```python
from build123d import *

# Parameters (mm, degrees)
SKETCH2_R           = 60
BOSS_EXTRUDE2_DEPTH = 5


with BuildPart() as part:
    # Sketch2 → Boss-Extrude2 (new body)
    with BuildSketch(Plane(origin=(0, 0, 0), x_dir=(0, 0, -1), z_dir=(1, 0, 0))):
        Circle(SKETCH2_R)
        with BuildLine():
            Line((-32.360679775, 14.767876284), (-44.805880919, 31.897226135))
            ThreePointArc((-44.805880919, 31.897226135), (-32.328188876, 44.495934691), (-16.490286116, 52.469709965))
            Line((-16.490286116, 52.469709965), (-4.045084972, 35.340360114))
            Line((-4.045084972, 35.340360114), (-32.360679775, 14.767876284))
        make_face(mode=Mode.SUBTRACT)
        with BuildLine():
            Line((-47.702148851, 27.37708887), (-36.405764747, 11.828950023))
            Line((-36.405764747, 11.828950023), (-55, 0))
            ThreePointArc((-55, 0), (-53.144229164, 14.166541801), (-47.702148851, 27.37708887))
        make_face(mode=Mode.SUBTRACT)
        with BuildLine():
            Line((0, 38.279286376), (-11.296384104, 53.827425223))
            ThreePointArc((-11.296384104, 53.827425223), (0, 55), (11.296384104, 53.827425223))
            Line((11.296384104, 53.827425223), (0, 38.279286376))
        make_face(mode=Mode.SUBTRACT)
        with BuildLine():
            Line((-54.718344288, -5.559028547), (-34.860679775, 7.073667441))
            Line((-34.860679775, 7.073667441), (-24.045084972, -26.213310629))
            Line((-24.045084972, -26.213310629), (-44.181843419, -32.756140067))
            ThreePointArc((-44.181843419, -32.756140067), (-51.285792388, -19.868756859), (-54.718344288, -5.559028547))
        make_face(mode=Mode.SUBTRACT)
        with BuildLine():
            Line((4.045084972, 35.340360114), (16.490286116, 52.469709965))
            ThreePointArc((16.490286116, 52.469709965), (32.328188876, 44.495934691), (44.805880919, 31.897226135))
            Line((44.805880919, 31.897226135), (32.360679775, 14.767876284))
            Line((32.360679775, 14.767876284), (4.045084972, 35.340360114))
        make_face(mode=Mode.SUBTRACT)
        with BuildLine():
            Line((-40.77793343, -36.907453789), (-22.5, -30.968593211))
            Line((-22.5, -30.968593211), (-22.5, -50.18714975))
            ThreePointArc((-22.5, -50.18714975), (-32.328188876, -44.495934691), (-40.77793343, -36.907453789))
        make_face(mode=Mode.SUBTRACT)
        with BuildLine():
            Line((36.405764747, 11.828950023), (47.702148851, 27.37708887))
            ThreePointArc((47.702148851, 27.37708887), (52.308108396, 16.995934691), (54.683698177, 5.890089445))
            Line((54.683698177, 5.890089445), (36.405764747, 11.828950023))
        make_face(mode=Mode.SUBTRACT)
        with BuildLine():
            Line((-17.5, -52.141634037), (-17.5, -30.968593211))
            Line((-17.5, -30.968593211), (17.5, -30.968593211))
            Line((17.5, -30.968593211), (17.5, -52.141634037))
            ThreePointArc((17.5, -52.141634037), (0, -55), (-17.5, -52.141634037))
        make_face(mode=Mode.SUBTRACT)
        with BuildLine():
            Line((34.860679775, 7.073667441), (54.997438222, 0.530838003))
            ThreePointArc((54.997438222, 0.530838003), (52.308108396, -16.995934691), (44.181843419, -32.756140067))
            Line((44.181843419, -32.756140067), (24.045084972, -26.213310629))
            Line((24.045084972, -26.213310629), (34.860679775, 7.073667441))
        make_face(mode=Mode.SUBTRACT)
        with BuildLine():
            Line((22.5, -50.18714975), (22.5, -30.968593211))
            Line((22.5, -30.968593211), (40.77793343, -36.907453789))
            ThreePointArc((40.77793343, -36.907453789), (32.328188876, -44.495934691), (22.5, -50.18714975))
        make_face(mode=Mode.SUBTRACT)
        Polygon((-20.572949017, -25.764282653), (-31.787730758, 8.751266486), (-2.427050983, -0.788596668), align=None, mode=Mode.SUBTRACT)
        Polygon((18.145898034, -27.527638409), (-18.145898034, -27.527638409), (0, -2.551952425), align=None, mode=Mode.SUBTRACT)
        Polygon((31.787730758, 8.751266486), (20.572949017, -25.764282653), (2.427050983, -0.788596668), align=None, mode=Mode.SUBTRACT)
        Polygon((-30.860679775, 11.604436034), (-1.5, 32.936218542), (-1.5, 2.064572881), align=None, mode=Mode.SUBTRACT)
        Polygon((1.5, 32.936218542), (30.860679775, 11.604436034), (1.5, 2.064572881), align=None, mode=Mode.SUBTRACT)
    extrude(amount=BOSS_EXTRUDE2_DEPTH)


solid = part.part
```
Check sheet for the modelled part. Datum: model origin and axes. Units: mm. Coordinates: 2 decimals unless noted, no trailing zeros. Write each loop counter-clockwise with the first axis right and the second up, starting at its lowest first coordinate (ties: lowest second). Pieces come first, ordered by that corner, then holes. Notation, with made-up numbers: (-0.75, -36.75) -> (42.25, -36.75) arc R21 cw to (42.25, -17.75) -> close; hole circle Ø9 at (40.25, 88). An arc over 180 degrees is marked (long way). Use a Markdown table: item, result.
1. Sectioned sample at A-A (z = 15). Enter the section's corners in (x, y).
Reported:
| item | result |
|---|---|
| outline | (0, -58.09) -> (5, -58.09) -> (5, -52.92) -> (0, -52.92) -> close; (0, -30.97) -> (5, -30.97) -> (5, -27.53) -> (0, -27.53) -> close; (0, -23.2) -> (5, -23.2) -> (5, -18.09) -> (0, -18.09) -> close; (0, 3.3) -> (5, 3.3) -> (5, 6.45) -> (0, 6.45) -> close; (0, 23.13) -> (5, 23.13) -> (5, 27.38) -> (0, 27.38) -> close; (0, 50.42) -> (5, 50.42) -> (5, 58.09) -> (0, 58.09) -> close |
2. Sectioned sample at C-C (y = -15.5). Enter the section's corners in (x, z).
Reported:
| item | result |
|---|---|
| outline | (0, -57.96) -> (5, -57.96) -> (5, -52.77) -> (0, -52.77) -> close; (0, -27.53) -> (5, -27.53) -> (5, -23.91) -> (0, -23.91) -> close; (0, -13.12) -> (5, -13.12) -> (5, -9.41) -> (0, -9.41) -> close; (0, 9.41) -> (5, 9.41) -> (5, 13.12) -> (0, 13.12) -> close; (0, 23.91) -> (5, 23.91) -> (5, 27.53) -> (0, 27.53) -> close; (0, 52.77) -> (5, 52.77) -> (5, 57.96) -> (0, 57.96) -> close |
3. Sectioned sample at B-B (y = 29.5). Enter the section's corners in (x, z).
Reported:
| item | result |
|---|---|
| outline | (0, -52.25) -> (5, -52.25) -> (5, -43.06) -> (0, -43.06) -> close; (0, -12.08) -> (5, -12.08) -> (5, -6.23) -> (0, -6.23) -> close; (0, -1.5) -> (5, -1.5) -> (5, 1.5) -> (0, 1.5) -> close; (0, 6.23) -> (5, 6.23) -> (5, 12.08) -> (0, 12.08) -> close; (0, 43.06) -> (5, 43.06) -> (5, 52.25) -> (0, 52.25) -> close |
4. Release check for a two-part mould opening along Z. For faces 1 (the flat face through (5, 0, 0)), 2 (the flat face through (2, -42, 17.5)) record: pulls with the +Z half, pulls with the -Z half, needs draft (parallel to the pull), parting line crosses it, or undercut.
Reported:
| item | result |
|---|---|
| face 1 | needs draft |
| face 2 | undercut |
5. Sectioned sample at D-D (x = 1). Give the number of separate pieces and of enclosed holes in the cut face, plus the area to 3 significant figures.
Reported:
| item | result |
|---|---|
| separate pieces | 1 |
| enclosed holes | 15 |
| area | 4,050 mm2 |
6. Go/stop test with flat-tipped pins: pin 1 Ø1.5 at (x, z) = (2.5, -1.5) entering from -Y; pin 2 Ø1.5 at (x, y) = (2.5, -39.5) entering from +Z; pin 3 Ø1.5 at (x, y) = (3, 21.5) entering from -Z. Record where each tip stops, or that it passes through.
Reported:
| item | result |
|---|---|
| pin 1 | stops at y = -60 |
| pin 2 | stops at z = 45.81 |
| pin 3 | stops at z = -56.3 |
7. Scan lines: line 1 along Y through (x, z) = (1.2, -20); line 2 along Y through (x, z) = (4.4, 44.5); line 3 along Z through (x, y) = (3.3, -18.5). Record each from-to range of solid material in increasing order.
Reported:
| item | result |
|---|---|
| line 1 | y = -56.57 to -24.98, 4.92 to 8.08, 19.5 to 23.75, 51.23 to 56.57 |
| line 2 | y = -40.25 to -32.32, 0.94 to 6.68, 22.97 to 31.48, 32.32 to 40.25 |
| line 3 | z = -57.08 to -51.8, -26.55 to -22.93, -15.3 to -11.59, 11.59 to 15.3, 22.93 to 26.55, 51.8 to 57.08 |
